```python
from build123d import *

# Parameters (mm, degrees)
F1_DEPTH = 6.35
F2_R     = 1.5
F2_R_2   = 1.6
F3_DEPTH = 6.351
F5_DEPTH = 3
F6_R     = 2.99999


# Not quite as in the source:
# - a fillet or chamfer is up to 0.001 mm smaller than in the source, because OpenCascade refuses the exact size


with BuildPart() as f1:
    # F0 (on Front) → F1 (new body)
    with BuildSketch(Plane.XZ):
        with BuildLine():
            Line((33, 6.3125771578), (-19, 6.3125771578))
            ThreePointArc((-19, 6.3125771578), (-21.1213203436, 5.4338975014), (-22, 3.3125771578))
            Line((-22, 3.3125771578), (-22, -2.6874228422))
            ThreePointArc((-22, -2.6874228422), (-21.1213203436, -4.8087431858), (-19, -5.6874228422))
            Line((-19, -5.6874228422), (33, -5.6874228422))
            Line((33, -5.6874228422), (33, -18.461904466))
            Line((33, -18.461904466), (33, -26.461904466))
            Line((33, -26.461904466), (34.9491434073, -32.6615871174))
            ThreePointArc((34.9491434073, -32.6615871174), (38.7515149865, -35.4618817353), (42.5726810332, -32.6872881404))
            Line((42.5726810332, -32.6872881404), (44.5761270821, -26.461904466))
            Line((44.5761270821, -26.461904466), (44.5761270821, -18.461904466))
            Line((44.5761270821, -18.461904466), (44.5761270821, 1.3125771578))
            ThreePointArc((44.5761270821, 1.3125771578), (43.111660988, 4.8481110637), (39.5761270821, 6.3125771578))
            Line((39.5761270821, 6.3125771578), (33, 6.3125771578))
        make_face()
    extrude(amount=F1_DEPTH)

    # F2 (on face) → F3 (cut, through all)
    with BuildSketch(Plane.XZ):
        with Locations((-15, 0)):
            Circle(F2_R)
        with Locations((15, 0)):
            Circle(F2_R)
        with Locations((38.765, -13.461904466)):
            Circle(F2_R_2)
        with Locations((38.765, -31.461904466)):
            Circle(F2_R_2)
    extrude(amount=F3_DEPTH, mode=Mode.SUBTRACT)

    # F4 (on face) → F5 (join)
    with BuildSketch(Plane.XZ):
        Polygon((41.4565890705, -5.352164329), (32.2204606053, 2.3090321163), (30.305161494, 0), (39.5412899592, -7.6611964453), align=None)
    extrude(amount=-F5_DEPTH)

    # F6 (radius 3 in the source; OpenCascade refuses exactly that, so slightly less here)
    f6_edges = [f1.edges().sort_by_distance(p)[0] for p in [
        (31.262811, 3, 1.154516),
        (40.49894, 3, -6.50668),
    ]]
    fillet(f6_edges, radius=F6_R)


solid = f1.part
```
CAD build for the part. Positions are in the model's coordinates, mm. A direction names the side the tool comes from. Round coordinates to 2 decimals unless told otherwise and drop trailing zeros. Write each loop counter-clockwise with the first axis right and the second up, starting at its lowest first coordinate (ties: lowest second). Pieces come first, ordered by that corner, then holes. Notation, with made-up numbers: M 79,78 L 96,78 A25 cw 96,108 Z; hole C 38.5,-36.75 d2. An arc over 180 degrees is marked long. One line per question, with ' | ' between items.
1. Cut at D-D on x = -1.5. Write the cut outline in (y, z).
Working result:
outline: M -6.35,-5.69 L 0,-5.69 L 0,6.31 L -6.35,6.31 Z
2. Mould opens along Z. For faces 1 (the flat face through (-22, -3, 0)), 2 (the cylindrical face through (-16.5, -3.13, 0.07)), 3 (the cylindrical face through (-21.14, -3.13, -4.79)) say: pulls with the +Z half, pulls with the -Z half, needs draft (parallel to the pull), parting line crosses it, or undercut.
Working result:
face 1: needs draft | face 2: undercut | face 3: pulls with the -Z half
3. Cut at C-C on z = -9.5. Write the cut outline in (x, y), and give its area (3 significant figures).
Working result:
outline: M 33,-6.35 L 44.58,-6.35 L 44.58,0 L 33,0 Z | area: 73.5 mm2
4. Cut at A-A on x = 15. Write the cut outline in (y, z).
Working result:
outline: M -6.35,-5.69 L 0,-5.69 L 0,-1.5 L -6.35,-1.5 Z; M -6.35,1.5 L 0,1.5 L 0,6.31 L -6.35,6.31 Z
5. Probe L1, parallel to X at y = -1.5, z = 0; L2, parallel to Z at x = -15, y = -3; L3, parallel to X at y = -4.75, z = -18.5. List the from-to ranges inside material, lowest first. Write a range as from..to.
Working result:
L1: -22..-16.5, -13.5..13.5, 16.5..44.58 | L2: -5.69..-1.5, 1.5..6.31 | L3: 33..44.58
6. Pin check, flat tips, straight feed: pin 1 Ø1.8 at (x, z) = (-15, 0) entering from -Y; pin 2 Ø5 at (x, z) = (15, 0) entering from -Y; pin 3 Ø3 at (y, z) = (-2, -19.5) entering from -X; pin 4 Ø5 at (x, y) = (10.5, -4) entering from -Z. Stop position of each tip, or through.
Working result:
pin 1: through | pin 2: y = -6.35 | pin 3: x = 33 | pin 4: z = -5.69
7. Cut at B-B on y = -1. Write the cut outline in (x, z) (3 decimals).
Working result:
outline: M -22,-2.687 A3 ccw -19,-5.687 L 33,-5.687 L 33,-26.462 L 34.949,-32.662 A4 ccw 42.573,-32.687 L 44.576,-26.462 L 44.576,1.313 A5 ccw 39.576,6.313 L -19,6.313 A3 ccw -22,3.313 Z; hole C -15,0 d3; hole C 15,0 d3; hole C 38.765,-31.462 d3.2; hole C 38.765,-13.462 d3.2
8. Which spindle directions (+Z, -Z, +X, -X, +Y, -Y) get a long thin tool onto all of the face, cutting with end or side? Do faces 4 (the cylindrical face through (13.5, -3.13, 0.07)), 5 (the flat face through (34.86, 1.48, -3.78)), 6 (the flat face through (33, -3, -16)), 7 (the flat face through (36.903, 1.479, -1.575)). Say none if no direction does.
Working result:
face 4: +Y, -Y | face 5: -Z, -X, +Y | face 6: -Z, -X, +Y, -Y | face 7: +Z, +X, +Y
